The listing builds one solid part. Answer for the finished solid, in the listing's coordinates (mm). A direction names the side the tool comes from. Round coordinates to 2 decimals unless told otherwise and drop trailing zeros. Write each loop counter-clockwise with the first axis right and the second up, starting at its lowest first coordinate (ties: lowest second). Pieces come first, ordered by that corner, then holes. Notation, with made-up numbers: M 40.5,-0.75 L 91.5,-0.75 A20 ccw 91.5,35.25 Z; hole C 80,41 d10. An arc over 180 degrees is marked long. One line per item, written item: value. Start each with the question number.
(1) Consider probe 1 along Z at (x, y) = (33.25, -2.5) (3 decimals); probe 2 along X at (y, z) = (3, 0.9); probe 3 along X at (y, z) = (2.75, 3.15). Determine where each line is inside the solid, lowest interval first.
(2) For faces 3 (the cylindrical face through (-33.444, -2.455, 3.024)), 4 (the cylindrical face through (33.444, -2.455, 0.976)), 5 (the cylindrical face through (23.526, -1.019, 3.113)), 6 (the cylindrical face through (-17.6, -1.4, 1.1)), determine the directions among +Z, -Z, +X, -X, +Y, -Y from which every point of the face is accessible in a straight line to the end or side of a thin tool.
(3) Given P1, Ø3, axis at x = -7, y = 2.5, coming from the -Z side; P2, Ø3.5, axis at x = -20.5, y = -1.5, coming from the -Z side; P3, Ø3, axis at x = -23.5, y = 3, coming from the -Z side, each flat-ended and moving along its own axis, determine where each tip first touches the part or whether it passes through.
(4) For a pull along Y with two mould halves and no side action, classify faces 1 (the conical face through (-28.99, -2.67, 1.96)), 2 (the flat face through (-37.5, 0, 2)) as released by +Y, released by -Y, zero draft, split by the parting line, or undercut.
(5) Section B-B (x = -20.5) is taken. Determine the outline of the cut face in (y, z), plus the area to 3 significant figures.
(6) Section A-A (x = -13) is taken. Determine the outline of the cut face in (y, z), plus the area to 3 significant figures.
```python
from build123d import *

# Parameters (mm, degrees)
SKETCH1_W                                        = 75
SKETCH1_H                                        = 10
BOSS_EXTRUDE1_DEPTH                              = 4
F_2_5_2_5_DIAMETER_HOLE1_D                       = 2.5
F_2_5_2_5_DIAMETER_HOLE1_DEPTH                   = 4
CBORE_FOR_M3_HEX_HEAD_MACHINE_SCREW1_D           = 3.2
CBORE_FOR_M3_HEX_HEAD_MACHINE_SCREW1_DEPTH       = 4
CBORE_FOR_M3_HEX_HEAD_MACHINE_SCREW1_CBORE_D     = 5.8
CBORE_FOR_M3_HEX_HEAD_MACHINE_SCREW1_CBORE_DEPTH = 2.2
CBORE_FOR_M2_HEX_HEAD_MACHINE_SCREW1_D           = 2.2
CBORE_FOR_M2_HEX_HEAD_MACHINE_SCREW1_DEPTH       = 4
CBORE_FOR_M2_HEX_HEAD_MACHINE_SCREW1_CBORE_D     = 4.499999997
CBORE_FOR_M2_HEX_HEAD_MACHINE_SCREW1_CBORE_DEPTH = 1.6
F_2_05_2_05_DIAMETER_HOLE1_D                     = 2.05
F_2_05_2_05_DIAMETER_HOLE1_DEPTH                 = 8
F_2_05_2_05_DIAMETER_HOLE1_TIP                   = 0.615882135
F_2_05_2_05_DIAMETER_HOLE2_D                     = 2.05
F_2_05_2_05_DIAMETER_HOLE2_DEPTH                 = 8
F_2_05_2_05_DIAMETER_HOLE2_TIP                   = 0.615882135


with BuildPart() as part:
    # Sketch1 → Boss-Extrude1 (new body)
    with BuildSketch(Plane.XY.offset(4)):
        Rectangle(SKETCH1_W, SKETCH1_H)
    extrude(amount=-BOSS_EXTRUDE1_DEPTH)

    # Ø2.5 (2.5) Diameter Hole1
    with Locations(Plane(origin=(0, 0, 0), x_dir=(-1, 0, 0), z_dir=(0, 0, -1))):
        with Locations((-13, -2), (13, -2)):
            Hole(F_2_5_2_5_DIAMETER_HOLE1_D / 2, depth=F_2_5_2_5_DIAMETER_HOLE1_DEPTH)

    # CBORE for M3 Hex Head Machine Screw1
    with Locations(Plane(origin=(0, 0, 0), x_dir=(-1, 0, 0), z_dir=(0, 0, -1))):
        with Locations((-22, -1.5), (20.5, -1.5)):
            CounterBoreHole(CBORE_FOR_M3_HEX_HEAD_MACHINE_SCREW1_D / 2, CBORE_FOR_M3_HEX_HEAD_MACHINE_SCREW1_CBORE_D / 2, CBORE_FOR_M3_HEX_HEAD_MACHINE_SCREW1_CBORE_DEPTH, depth=CBORE_FOR_M3_HEX_HEAD_MACHINE_SCREW1_DEPTH)

    # CBORE for M2 Hex Head Machine Screw1
    with Locations(Plane(origin=(0, 0, 0), x_dir=(-1, 0, 0), z_dir=(0, 0, -1))):
        with Locations((23.5, 3), (-25, 3)):
            CounterBoreHole(CBORE_FOR_M2_HEX_HEAD_MACHINE_SCREW1_D / 2, CBORE_FOR_M2_HEX_HEAD_MACHINE_SCREW1_CBORE_D / 2, CBORE_FOR_M2_HEX_HEAD_MACHINE_SCREW1_CBORE_DEPTH, depth=CBORE_FOR_M2_HEX_HEAD_MACHINE_SCREW1_DEPTH)

    # Ø2.05 (2.05) Diameter Hole1
    with Locations(Plane(origin=(37.5, 0, 0), x_dir=(0, 0, -1), z_dir=(1, 0, 0))):
        with Locations((-2, 2.5), (-2, -2.5)):
            Hole(F_2_05_2_05_DIAMETER_HOLE1_D / 2, depth=F_2_05_2_05_DIAMETER_HOLE1_DEPTH)
            with Locations((0, 0, -(F_2_05_2_05_DIAMETER_HOLE1_DEPTH + F_2_05_2_05_DIAMETER_HOLE1_TIP / 2))):  # 118° drill point
                Cone(0, F_2_05_2_05_DIAMETER_HOLE1_D / 2, F_2_05_2_05_DIAMETER_HOLE1_TIP, mode=Mode.SUBTRACT)

    # Ø2.05 (2.05) Diameter Hole2
    with Locations(Plane.ZY.offset(37.5)):
        with Locations((2, -2.5), (2, 2.5)):
            Hole(F_2_05_2_05_DIAMETER_HOLE2_D / 2, depth=F_2_05_2_05_DIAMETER_HOLE2_DEPTH)
            with Locations((0, 0, -(F_2_05_2_05_DIAMETER_HOLE2_DEPTH + F_2_05_2_05_DIAMETER_HOLE2_TIP / 2))):  # 118° drill point
                Cone(0, F_2_05_2_05_DIAMETER_HOLE2_D / 2, F_2_05_2_05_DIAMETER_HOLE2_TIP, mode=Mode.SUBTRACT)


solid = part.part
```
Recorded:
1. probe 1: z = 0 to 0.975, 3.025 to 4
1. probe 2: x = -37.5 to -25.75, -21.25 to 22.75, 27.25 to 37.5
1. probe 3: x = -37.5 to -24.57, -22.43 to 23.93, 26.07 to 37.5
2. face 3: -X
2. face 4: +X
2. face 5: +Z, -Z
2. face 6: -Z
3. P1: stops at z = 0
3. P2: stops at z = 2.2
3. P3: stops at z = 1.6
4. face 1: undercut
4. face 2: zero draft
5. outline: M -5,0 L -4.4,0 L -4.4,2.2 L -3.1,2.2 L -3.1,4 L -5,4 Z; M 0.1,2.2 L 1.4,2.2 L 1.4,0 L 5,0 L 5,4 L 0.1,4 Z
5. area: 21.5 mm2
6. outline: M -5,0 L -3.25,0 L -3.25,4 L -5,4 Z; M -0.75,0 L 5,0 L 5,4 L -0.75,4 Z
6. area: 30.0 mm2
